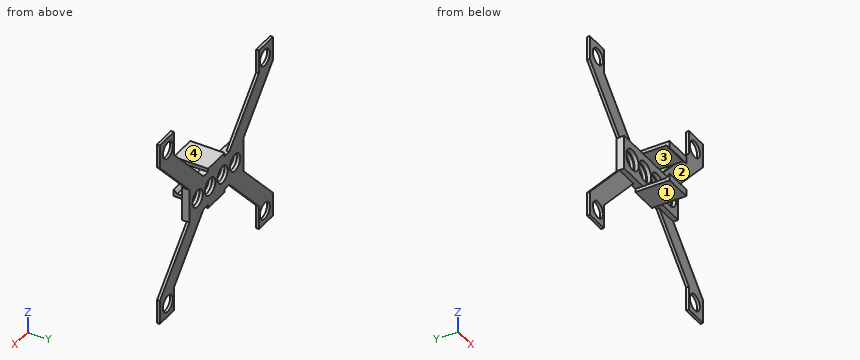
```python
from build123d import *

# Parameters (mm, degrees)
SKICA1_W                 = 26
SKICA1_H                 = 1
P_IDAT_VYSUNUT_M1_DEPTH  = 10
SKICA2_R                 = 2.5
ODEBRAT_VYSUNUT_M1_DEPTH = 1
SKICA3_R                 = 2.4
P_IDAT_VYSUNUT_M2_DEPTH  = 0.8
SKICA4_W                 = 26
SKICA4_H                 = 10
SKICA4_R                 = 3
P_IDAT_VYSUNUT_M3_DEPTH  = 1.2
SKICA6_W                 = 8
SKICA6_H                 = 1
P_IDAT_VYSUNUT_M5_DEPTH  = 10
P_IDAT_VYSUNUT_M6_DEPTH  = 8


with BuildPart() as part:
    # Skica1 → Přidat vysunutím1 (new body)
    with BuildSketch(Plane.XY):
        with Locations((-39.156744291, -7.214704976)):
            Rectangle(SKICA1_W, SKICA1_H)
    extrude(amount=P_IDAT_VYSUNUT_M1_DEPTH)

    # Skica2 → Odebrat vysunutím1 (cut)
    with BuildSketch(Plane(origin=(0, -7.714704976, 0), x_dir=(-1, 0, 0), z_dir=(0, -1, 0))):
        with Locations((48.186744291, -5)):
            Circle(SKICA2_R)
        with Locations((42.176744291, -5)):
            Circle(SKICA2_R)
        with Locations((36.166744291, -5)):
            Circle(SKICA2_R)
        with Locations((30.156744291, -5)):
            Circle(SKICA2_R)
    extrude(amount=-ODEBRAT_VYSUNUT_M1_DEPTH, mode=Mode.SUBTRACT)

    # Skica3 → Přidat vysunutím2 (add)
    with BuildSketch(Plane(origin=(0, -6.714704976, 0), x_dir=(1, 0, 0), z_dir=(0, 1, 0))):
        Polygon((-32.956744291, 0), (-18.656744291, 15.3), (-18.656744291, 22.3), (-11.856744291, 22.3), (-11.856744291, 15.3), (-26.156744291, 0), align=None)
        with Locations((-15.756744291, 18.4)):
            Circle(SKICA3_R, mode=Mode.SUBTRACT)
        Polygon((-52.156744291, 0), (-45.356744291, 0), (-59.656744291, 15.3), (-59.656744291, 22.3), (-66.456744291, 22.3), (-66.456744291, 15.3), align=None)
        with Locations((-62.556744291, 18.4)):
            Circle(SKICA3_R, mode=Mode.SUBTRACT)
        Polygon((-45.356744291, -10), (-59.656744291, -25.3), (-59.656744291, -32.3), (-66.456744291, -32.3), (-66.456744291, -25.3), (-52.156744291, -10), align=None)
        with Locations((-62.556744291, -28.4)):
            Circle(SKICA3_R, mode=Mode.SUBTRACT)
        Polygon((-26.156744291, -10), (-32.956744291, -10), (-18.656744291, -25.3), (-18.656744291, -32.3), (-11.856744291, -32.3), (-11.856744291, -25.3), align=None)
        with Locations((-15.756744291, -28.4)):
            Circle(SKICA3_R, mode=Mode.SUBTRACT)
    extrude(amount=-P_IDAT_VYSUNUT_M2_DEPTH)

    # Skica4 → Přidat vysunutím3 (add)
    with BuildSketch(Plane(origin=(0, -7.714704976, 0), x_dir=(-1, 0, 0), z_dir=(0, -1, 0))):
        with Locations((39.156744291, -5)):
            Rectangle(SKICA4_W, SKICA4_H)
        with Locations((48.186744291, -5)):
            Circle(SKICA4_R, mode=Mode.SUBTRACT)
        with Locations((42.176744291, -5)):
            Circle(SKICA4_R, mode=Mode.SUBTRACT)
        with Locations((36.166744291, -5)):
            Circle(SKICA4_R, mode=Mode.SUBTRACT)
        with Locations((30.156744291, -5)):
            Circle(SKICA4_R, mode=Mode.SUBTRACT)
    extrude(amount=P_IDAT_VYSUNUT_M3_DEPTH)

    # Skica6 → Přidat vysunutím5 (add)
    with BuildSketch(Plane(origin=(0, -6.714704976, 0), x_dir=(1, 0, 0), z_dir=(0, 1, 0))):
        with Locations((-39.156744291, 0.5)):
            Rectangle(SKICA6_W, SKICA6_H)
        with Locations((-39.156744291, -10.5)):
            Rectangle(SKICA6_W, SKICA6_H)
    extrude(amount=-P_IDAT_VYSUNUT_M5_DEPTH)

    # Skica7 → Přidat vysunutím6 (add)
    with BuildSketch(Plane(origin=(-35.156744291, 0, 0), x_dir=(0, 0, -1), z_dir=(1, 0, 0))):
        Polygon((0, -16.714704976), (-1, -16.714704976), (0, -15.714704976), align=None)
        Polygon((-10, -16.714704976), (-9, -16.714704976), (-10, -15.714704976), align=None)
    extrude(amount=-P_IDAT_VYSUNUT_M6_DEPTH)


solid = part.part
```
Here's how the part is built. I have some questions about the finished solid (model axes, mm). Face numbers are marked on the shaded views. Coordinates: 2 decimals unless noted, no trailing zeros. Loops run counter-clockwise (first coordinate to the right, second up) from the corner with the lowest first, then second, coordinate; pieces in that order, holes last. Notation, with made-up numbers: (33, 0) -> (64, 0) arc R31 cw to (64, 29) -> close; hole circle Ø7 at (73.5, 44.25). An arc over 180 degrees is marked (long way). Return JSON: item names as keys, results as strings.
1) Will these pins go through, and if not, where does the flat tip stop? pin 1 (10.5 mm diameter, centred on x = -25.5, z = 17.5, fed in from -Y); pin 2 (5 mm diameter, centred on x = -37, z = 4, fed in from -Y); pin 3 (2 mm diameter, centred on y = -11.5, z = 10.5, fed in from +X).
Results below:
{"pin 1": "y = -7.51", "pin 2": "y = -8.91", "pin 3": "x = -35.16"}
2) If we section it at C-C, the plane x = -16.5: Write out the boundary of the cut face in (y, z).
Results below:
{"outline": "(-7.51, -22.3) -> (-6.71, -22.3) -> (-6.71, -20.68) -> (-7.51, -20.68) -> close; (-7.51, -16.12) -> (-6.71, -16.12) -> (-6.71, -10.33) -> (-7.51, -10.33) -> close; (-7.51, 20.33) -> (-6.71, 20.33) -> (-6.71, 26.12) -> (-7.51, 26.12) -> close; (-7.51, 30.68) -> (-6.71, 30.68) -> (-6.71, 32.3) -> (-7.51, 32.3) -> close"}
3) If we section it at D-D, the plane z = 17.5: Write out the boundary of the cut face in (x, y), then the cut area to 3 significant figures.
Results below:
{"outline": "(-59.17, -7.51) -> (-52.37, -7.51) -> (-52.37, -6.71) -> (-59.17, -6.71) -> close; (-25.95, -7.51) -> (-19.15, -7.51) -> (-19.15, -6.71) -> (-25.95, -6.71) -> close", "area": "10.9 mm²"}
4) Thinking about a two-plate mould opening in Z: for the marked faces 1, 2, 3 and 4, which applies, +Z half, -Z half, draft (parallel to the pull), parting line (faces both ways), or undercut?
Results below:
{"face 1": "-Z half", "face 2": "draft", "face 3": "undercut", "face 4": "+Z half"}
5) If we section it at B-B, the plane z = -18.4: Write out the boundary of the cut face in (x, y).
Results below:
{"outline": "(-66.46, -7.51) -> (-64.96, -7.51) -> (-64.96, -6.71) -> (-66.46, -6.71) -> close; (-60.16, -7.51) -> (-59.66, -7.51) -> (-59.66, -6.71) -> (-60.16, -6.71) -> close; (-18.66, -7.51) -> (-18.16, -7.51) -> (-18.16, -6.71) -> (-18.66, -6.71) -> close; (-13.36, -7.51) -> (-11.86, -7.51) -> (-11.86, -6.71) -> (-13.36, -6.71) -> close"}
6) If we section it at A-A, the plane y = -14.25: Write out the boundary of the cut face in (x, z), then the cut area to 3 significant figures.
Results below:
{"outline": "(-43.16, -1) -> (-35.16, -1) -> (-35.16, 0) -> (-43.16, 0) -> close; (-43.16, 10) -> (-35.16, 10) -> (-35.16, 11) -> (-43.16, 11) -> close", "area": "16.0 mm²"}
7) I need wall thicknesses on line 1 (X direction, y = -7.5, z = 5); line 2 (X direction, y = -7.05, z = -18.4); line 3 (Z direction, x = -36, y = -9.75). Which ranges of each line are inside material? Lowest first, please. Write a range as from..to.
Results below:
{"line 1": "-52.16..-50.69, -45.69..-44.68, -39.68..-38.67, -33.67..-32.66, -27.66..-26.16", "line 2": "-66.46..-64.96, -60.16..-59.66, -18.66..-18.16, -13.36..-11.86", "line 3": "-1..0, 10..11"}
